Can you work these out from the model? Positions are in its coordinate system, mm. Face numbers are marked on the shaded views. A direction names the side the tool comes from. Give positions to 0.01 mm unless a question says otherwise; leave off trailing zeros. Loops run counter-clockwise (first coordinate to the right, second up) from the corner with the lowest first, then second, coordinate; pieces in that order, holes last.
from build123d import *


with BuildPart() as part:
    # Body Sketch → Body Revolve (revolve)
    with BuildSketch(Plane(origin=(0, 0, 0), x_dir=(1, 0, 0), z_dir=(0, 1, 0)), mode=Mode.PRIVATE) as body_revolve_sk:
        Polygon((2.65, -14.75), (3.1, -14.75), (3.1, -12.25), (5.225, -12.25), (5.225, -11.25), (3.1, -11.25), (3.1, -5.95), (1.625, -5.55), (1.625, -4.15), (2.5, -4.15), (2.5, -3.4), (0.25, -3.4), (0.25, -5.954207714), (2.65, -6.605055172), align=None)
    revolve(body_revolve_sk.sketch.rotate(Axis((0, 0, 0), (0, 0, 1)), 180), axis=Axis((0, 0, 0), (0, 0, 1)))

    # N08 Sketch → N08 Revolve (revolve)
    with BuildSketch(Plane(origin=(0, 0, 0), x_dir=(1, 0, 0), z_dir=(0, 1, 0)), mode=Mode.PRIVATE) as n08_revolve_sk:
        Polygon((0.5, 0), (0.75, 0), (0.75, -0.75), (1.25, -3.4), (0.5, -3.4), align=None)
    revolve(n08_revolve_sk.sketch.rotate(Axis((0, 0, 0), (0, 0, 1)), 180), axis=Axis((0, 0, 0), (0, 0, 1)))


solid = part.part
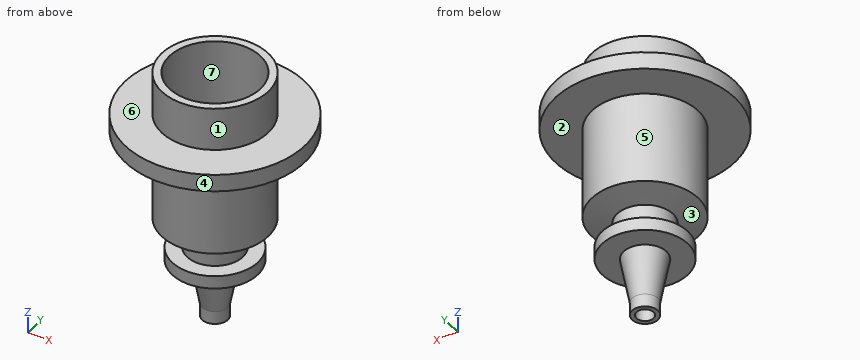
(1) Suppose I cut it at D-D on y = 3.5. List the corners of the cut face in (x, z) for me, plus the area to 3 significant figures.
Returned:
outline: (-3.88, 11.25) - (3.88, 11.25) - (3.88, 12.25) - (-3.88, 12.25) - close
area: 7.76 mm2
(2) Which directions (+Z, -Z, +X, -X, +Y, -Y) give clear straight access to the entire face, cutting with the end or side of a thin tool? Please do the marked faces 1, 2, 3 and 4.
Returned:
face 1: +Z
face 2: -Z
face 3: none
face 4: +Z, -Z
(3) Suppose I cut it at B-B on z = 4.5. List the corners of the cut face in (x, y) for me (3 decimals).
Returned:
outline: circle Ø3.25 at (0, 0); hole circle Ø0.5 at (0, 0)
(4) Please list where these lines run through material, in increasing order: probe 1 along Y at (x, z) = (0, 4.1); probe 2 along Y at (x, z) = (0, 7.75); probe 3 along Z at (x, y) = (-1.25, 4).
Returned:
probe 1: y = -2.5 to -0.25, 0.25 to 2.5
probe 2: y = -3.1 to -2.65, 2.65 to 3.1
probe 3: z = 11.25 to 12.25
(5) Suppose I cut it at C-C on y = -4.25. List the corners of the cut face in (x, z) for me.
Returned:
outline: (-3.04, 11.25) - (3.04, 11.25) - (3.04, 12.25) - (-3.04, 12.25) - close
(6) Suppose I cut it at A-A on z = 13.75. List the corners of the cut face in (x, y) for me.
Returned:
outline: circle Ø6.2 at (0, 0); hole circle Ø5.3 at (0, 0)
(7) Thinking about a two-plate mould opening in X: for the marked faces 5, 6 and 7, which applies, pulls with the +X half, pulls with the -X half, needs draft (parallel to the pull), parting line crosses it, or undercut?
Returned:
face 5: parting line crosses it
face 6: needs draft
face 7: undercut
(8) Will these pins go through, and if not, where does the flat tip stop? P1, Ø5, axis at x = 0.5, y = -0.5, coming from the -Z side; P2, Ø3, axis at y = 0, z = 6, coming from the -X side; P3, Ø0.8, axis at x = 0, y = 0, coming from the -Z side; P4, Ø1.5, axis at y = -2, z = 3.5, coming from the +X side.
Returned:
P1: stops at z = 0
P2: stops at x = -3.1
P3: stops at z = 3.4
P4: stops at x = 2.17
